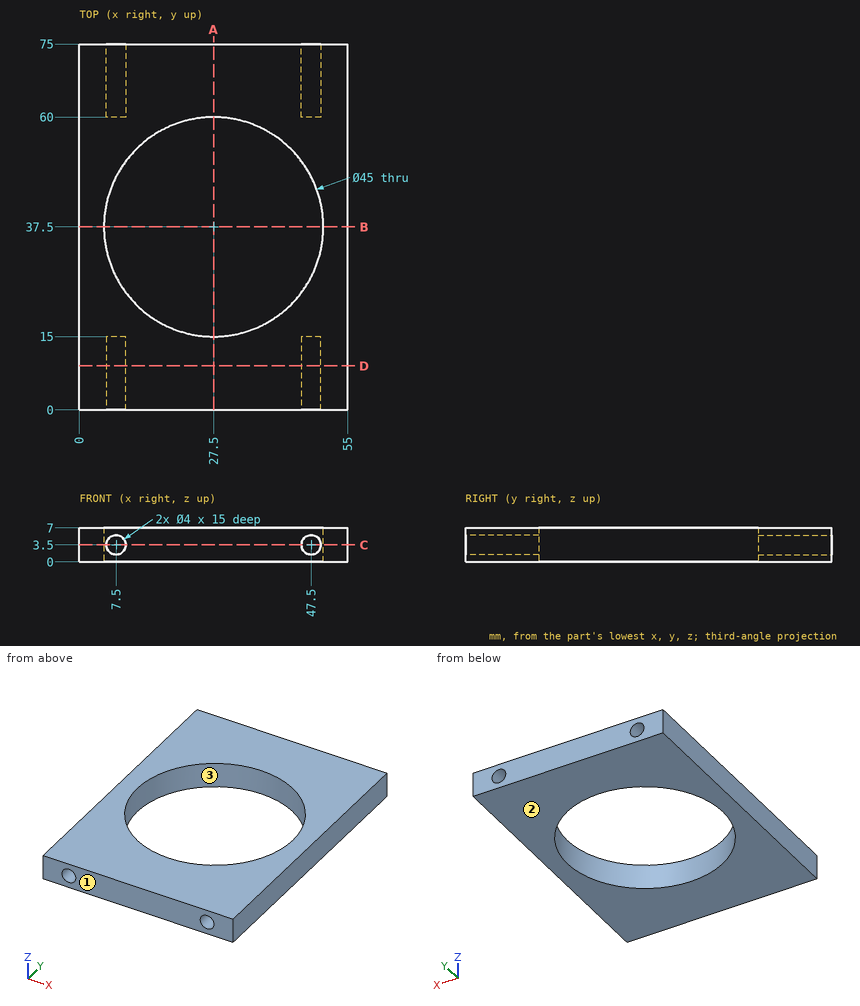
Source: three-view drawing plus pictorial views. Frame: mm from the lowest corner of the part. Give positions to 0.01 mm unless a question says otherwise; leave off trailing zeros. Write each loop counter-clockwise with the first axis right and the second up, starting at its lowest first coordinate (ties: lowest second). Pieces come first, ordered by that corner, then holes.
(1) Ray query, line 1 (Z direction, x = 47.5, y = 71); line 2 (X direction, y = 67.5, z = 3.5); line 3 (X direction, y = 6.5, z = 2.25). Return the intervals inside material, ascending.
(2) Cut plane C-C, the plane z = 3.5. Return loops of the section in (x, y).
(3) Cut plane D-D, the plane y = 9. Return loops of the section in (x, z).
(4) Cut plane B-B, the plane y = 37.5. Return loops of the section in (x, z).
(5) Mould query, pull axis Y, two halves, no side actions, for the marked faces 1, 2 and 3. Classes: released by +Y, released by -Y, zero draft, split by the parting line, or undercut.
(6) First-contact query: P1, Ø2.5, axis at x = 47.5, z = 3.5, coming from the +Y side; P2, Ø1.2, axis at x = 46.5, z = 3.5, coming from the -Y side; P3, Ø2, axis at x = 30, z = 6, coming from the -Y side. Flat tips, straight axial feed; report the tip coordinate or a pass-through.
(7) Cut plane A-A, the plane x = 27.5. Return loops of the section in (y, z), then the cut area to 3 significant figures.
Values follow:
1. line 1: z = 0 to 1.5, 5.5 to 7
1. line 2: x = 0 to 5.5, 9.5 to 45.5, 49.5 to 55
1. line 3: x = 0 to 5.94, 9.06 to 45.94, 49.06 to 55
2. outline: (0, 0) - (5.5, 0) - (5.5, 15) - (9.5, 15) - (9.5, 0) - (45.5, 0) - (45.5, 15) - (49.5, 15) - (49.5, 0) - (55, 0) - (55, 75) - (49.5, 75) - (49.5, 60) - (45.5, 60) - (45.5, 75) - (9.5, 75) - (9.5, 60) - (5.5, 60) - (5.5, 75) - (0, 75) - close; hole circle Ø45 at (27.5, 37.5)
3. outline: (0, 0) - (55, 0) - (55, 7) - (0, 7) - close; hole circle Ø4 at (7.5, 3.5); hole circle Ø4 at (47.5, 3.5)
4. outline: (0, 0) - (5, 0) - (5, 7) - (0, 7) - close; (50, 0) - (55, 0) - (55, 7) - (50, 7) - close
5. face 1: released by -Y
5. face 2: zero draft
5. face 3: undercut
6. P1: stops at y = 60
6. P2: stops at y = 15
6. P3: stops at y = 0
7. outline: (0, 0) - (15, 0) - (15, 7) - (0, 7) - close; (60, 0) - (75, 0) - (75, 7) - (60, 7) - close
7. area: 210 mm2
